Source: CAD feature listing. Evaluate the final solid. Frame: model axes, mm. Round coordinates to 2 decimals unless told otherwise and drop trailing zeros. Write each loop counter-clockwise with the first axis right and the second up, starting at its lowest first coordinate (ties: lowest second). Pieces come first, ordered by that corner, then holes.
```python
from build123d import *

# Parameters (mm, degrees)
SKETCH1_R           = 14.2875
BOSS_EXTRUDE1_DEPTH = 12.7


with BuildPart() as part:
    # Sketch1 → Boss-Extrude1 (new body, symmetric)
    with BuildSketch(Plane(origin=(0, 0, 0), x_dir=(0, 0, -1), z_dir=(1, 0, 0))):
        with BuildLine():
            Line((-38.1, 0), (38.1, 0))
            Line((38.1, 0), (38.1, 44.45))
            ThreePointArc((38.1, 44.45), (0, 82.55), (-38.1, 44.45))
            Line((-38.1, 44.45), (-38.1, 0))
        make_face()
        with Locations((0, 44.45)):
            Circle(SKETCH1_R, mode=Mode.SUBTRACT)
    extrude(amount=BOSS_EXTRUDE1_DEPTH, both=True)


solid = part.part
```
Q1. Mould query, pull axis Y, two halves, no side actions, for faces 1 (the face through (-0.178, 58.616, 1.86)), 2 (the face through (0, 0, 1)), 3 (the face through (0, 23, 38.1)). Classes: pulls with the +Y half, pulls with the -Y half, needs draft (parallel to the pull), parting line crosses it, or undercut.
Q2. Pin query (flat end, axial travel): P1, Ø1, axis at x = -9, z = -9, coming from the +Y side; P2, Ø23, axis at y = 44.45, z = 0, coming from the +X side; P3, Ø4, axis at x = -4, z = -12, coming from the +Y side. Return the tip coordinate at first contact, or that it passes through.
Q3. Section query A-A, the plane z = 0. Output: boundary loops of the cut face in (x, y), and give its area (3 significant figures).
Q4. Section query D-D, the plane z = -29. Output: boundary loops of the cut face in (x, y).
Q5. Section query B-B, the plane y = 51. Output: boundary loops of the cut face in (x, z).
Q6. Line query: line 1 (Y direction, x = 4.5, z = 0); line 2 (Z direction, x = 2, y = 50); line 3 (Y direction, x = -1, z = -3). Output: solid intervals per line, ascending.
Filled in:
1. face 1: undercut
1. face 2: pulls with the -Y half
1. face 3: needs draft
2. P1: stops at y = 81.59
2. P2: passes through
2. P3: stops at y = 81.21
3. outline: (-12.7, 0) - (12.7, 0) - (12.7, 30.16) - (-12.7, 30.16) - close; (-12.7, 58.74) - (12.7, 58.74) - (12.7, 82.55) - (-12.7, 82.55) - close
3. area: 1,370 mm2
4. outline: (-12.7, 0) - (12.7, 0) - (12.7, 69.16) - (-12.7, 69.16) - close
5. outline: (-12.7, -37.53) - (12.7, -37.53) - (12.7, -12.7) - (-12.7, -12.7) - close; (-12.7, 12.7) - (12.7, 12.7) - (12.7, 37.53) - (-12.7, 37.53) - close
6. line 1: y = 0 to 30.16, 58.74 to 82.55
6. line 2: z = -37.69 to -13.17, 13.17 to 37.69
6. line 3: y = 0 to 30.48, 58.42 to 82.43
